Solid Edge part; units mm, degrees
sketch "Sketch1" plane through (0, 0, 0) normal (0, 0, 1) x (1, 0, 0)
  line L0 (191, 107) -> (191, 86)
  line L1 (191, 86) -> (195, 86)
  line L2 (195, 86) -> (195, 107)
  line L3 (195, 107) -> (191, 107)
  line L4 (-195, -82) -> (-195, -102)
  line L5 (-195, -102) -> (-191, -102)
  line L6 (-191, -102) -> (-191, -82)
  line L7 (-191, -82) -> (-195, -82)
  line L8 (-195, 107) -> (-195, 86)
  line L9 (-195, 86) -> (-191, 86)
  line L10 (-191, 86) -> (-191, 107)
  line L11 (-191, 107) -> (-195, 107)
  line L12 (195, -82) -> (191, -82)
  line L13 (191, -82) -> (191, -102)
  line L14 (191, -102) -> (195, -102)
  line L15 (195, -102) -> (195, -82)
  line L16 (200, 115) -> (-200, 115)
  line L17 (-200, 115) -> (-200, -115)
  line L18 (-200, -115) -> (200, -115)
  line L19 (200, -115) -> (200, 115)
  line L20 (175, 90) -> (-175, 90)
  line L21 (-175, 90) -> (-175, -90)
  line L22 (-175, -90) -> (175, -90)
  line L23 (175, -90) -> (175, 90)
extrude "Protrusion1" add sketch "Sketch1" along normal blind 4
CAD build for the part. Positions are in the model's coordinates, mm. Coordinates: 2 decimals unless noted, no trailing zeros. Write each loop counter-clockwise with the first axis right and the second up, starting at its lowest first coordinate (ties: lowest second). Pieces come first, ordered by that corner, then holes. Notation, with made-up numbers: (-20, -9.75) - (17, -9.75) arc R19 cw to (17, 25.25) - close; hole circle Ø7 at (26.5, -3). An arc over 180 degrees is marked (long way). Use a Markdown table: item, result. Add a question column.
Item 1: Band-saw the part on A-A, the plane z = 1.2. Give the cut face in (x, y), and give its area (3 significant figures).
Item 2: Band-saw the part on B-B, the plane y = 96. Give the cut face in (x, z).
Item 3: Drill centre lines: L1, parallel to X at y = -98.5, z = 0.65; L2, parallel to Y at x = 107, z = 3.25; L3, parallel to X at y = -4, z = 2.25. Where is each one in solid material? Low to high. Write a range as from..to.
Item 4: Band-saw the part on D-D, the plane y = -37. Give the cut face in (x, z).
Item 5: Band-saw the part on C-C, the plane x = 66.5. Give the cut face in (y, z).
Numbers:
| question | item | result |
|---|---|---|
| 1 | outline | (-200, -115) - (200, -115) - (200, 115) - (-200, 115) - close; hole (-195, -102) - (-191, -102) - (-191, -82) - (-195, -82) - close; hole (-195, 86) - (-191, 86) - (-191, 107) - (-195, 107) - close; hole (-175, -90) - (175, -90) - (175, 90) - (-175, 90) - close; hole (191, -102) - (195, -102) - (195, -82) - (191, -82) - close; hole (191, 86) - (195, 86) - (195, 107) - (191, 107) - close |
| 1 | area | 28,700 mm2 |
| 2 | outline | (-200, 0) - (-195, 0) - (-195, 4) - (-200, 4) - close; (-191, 0) - (191, 0) - (191, 4) - (-191, 4) - close; (195, 0) - (200, 0) - (200, 4) - (195, 4) - close |
| 3 | L1 | -200..-195, -191..191, 195..200 |
| 3 | L2 | -115..-90, 90..115 |
| 3 | L3 | -200..-175, 175..200 |
| 4 | outline | (-200, 0) - (-175, 0) - (-175, 4) - (-200, 4) - close; (175, 0) - (200, 0) - (200, 4) - (175, 4) - close |
| 5 | outline | (-115, 0) - (-90, 0) - (-90, 4) - (-115, 4) - close; (90, 0) - (115, 0) - (115, 4) - (90, 4) - close |
